```python
from build123d import *

# Parameters (mm, degrees)
F_3_8_16_TAPPED_HOLE2_REACH  = 90.009
F_3_8_16_TAPPED_HOLE2_BORE_R = 3.96875
CIRPATTERN1_COUNT            = 6


with BuildPart() as part:
    # Sketch2 → Revolve1 (revolve)
    with BuildSketch(Plane.XY, mode=Mode.PRIVATE) as revolve1_sk:
        Polygon((-34.8996, 40.689305596), (-25.4, 40.689305596), (-25.4, 4.857627196), (-34.8996, 4.857627196), (-34.8996, 28.497305596), (-32.8676, 28.497305596), (-32.8676, 32.053305596), (-34.8996, 32.053305596), (-34.8996, 34.593305596), (-32.8676, 34.593305596), (-32.8676, 38.149305596), (-34.8996, 38.149305596), align=None)
    revolve(revolve1_sk.sketch.rotate(Axis((0, 0, 0), (0, 1, 0)), 270), axis=Axis((0, 0, 0), (0, 1, 0)))

    # 3/8-16 Tapped Hole2 bore → 3/8-16 Tapped Hole2 (cut, up to next)
    with BuildSketch(Plane(origin=(34.8996, 0, 0), x_dir=(0, 0, -1), z_dir=(1, 0, 0)), mode=Mode.PRIVATE) as f_3_8_16_tapped_hole2_sk1:
        with Locations((0, 17.372080196)):
            Circle(F_3_8_16_TAPPED_HOLE2_BORE_R)
    f_3_8_16_tapped_hole2_tool1 = extrude(f_3_8_16_tapped_hole2_sk1.sketch, amount=-F_3_8_16_TAPPED_HOLE2_REACH, mode=Mode.PRIVATE) & part.part
    f_3_8_16_tapped_hole2 = f_3_8_16_tapped_hole2_tool1.solids().sort_by_distance((34.8996, 17.37208, 0))[0]
    add(f_3_8_16_tapped_hole2, mode=Mode.SUBTRACT)

    # CirPattern1: 3/8-16 Tapped Hole2 ×6 about axis
    cirpattern1_axis = Axis((0, 40.689305596, 0), (0, -1, 0))
    for i in range(1, CIRPATTERN1_COUNT):
        add(f_3_8_16_tapped_hole2.rotate(cirpattern1_axis, i * 360 / CIRPATTERN1_COUNT), mode=Mode.SUBTRACT)


solid = part.part
```
Geometry check sheet. Reference: the model listing, model coordinates, mm. A direction names the side the tool comes from. Round coordinates to 2 decimals unless told otherwise and drop trailing zeros. Order: outer loops, then holes, each group sorted by start corner. A loop starts at its lowest first (then second) coordinate and runs counter-clockwise, first axis right, second up. Notation, with made-up numbers: M 38.25,-30 L 94.25,-30 A9 ccw 94.25,-17 Z; hole C 9.5,-39.75 d10. An arc over 180 degrees is marked long. Write item = value, one per line.
Q1. Scan lines: line 1 (Y direction, x = -26.75, z = 0); line 2 (Z direction, x = 30, y = 18); line 3 (Z direction, x = 17, y = 19.5). Record each from-to range of solid material in increasing order.
Answer block:
line_1 = 4.86 to 13.4, 21.34 to 40.69
line_2 = -17.83 to -3.92, 3.92 to 17.83
line_3 = -22.74 to -18.87, 18.87 to 22.74
Q2. Section check A-A (y = 16.5). Enter the section's corners in (x, z), plus the area to 3 significant figures.
Answer block:
outline = M -34.68,-3.87 A34.9 ccw -20.7,-28.1 L -15.9,-19.8 A25.4 cw -25.1,-3.87 Z; M -34.68,3.87 L -25.1,3.87 A25.4 cw -15.9,19.8 L -20.7,28.1 A34.9 ccw Z; M -13.99,-31.97 A34.9 ccw 13.99,-31.97 L 9.2,-23.68 A25.4 cw -9.2,-23.68 Z; M -13.99,31.97 L -9.2,23.68 A25.4 cw 9.2,23.68 L 13.99,31.97 A34.9 ccw Z; M 15.9,-19.8 L 20.7,-28.1 A34.9 ccw 34.68,-3.87 L 25.1,-3.87 A25.4 cw Z; M 15.9,19.8 A25.4 cw 25.1,3.87 L 34.68,3.87 A34.9 ccw 20.7,28.1 Z
area = 1,360 mm^2
Q3. Release check for a two-part mould opening along Y. For faces 3 (the cylindrical face through (-15.479, 21.307, 25.777)), 4 (the cylindrical face through (30.962, 33.341, -16.104)), 5 (the flat face through (26, 4.858, 2)), 6 (the flat face through (21, 38.149, 26)) record: released by +Y, released by -Y, zero draft, split by the parting line, or undercut.
Answer block:
face_3 = undercut
face_4 = zero draft
face_5 = released by -Y
face_6 = undercut
Q4. Set-up check for faces 1 (the cylindrical face through (-7.629, 22.523, -24.227)), 2 (the flat face through (26, 34.593, -21)): record each of +Z, -Z, +X, -X, +Y, -Y from which the full face is reachable in a straight line by a thin tool's end or side.
Answer block:
face_1 = +Y, -Y
face_2 = none
Q5. Depth check by flat-ended pin: pin 1 Ø1.5 at (y, z) = (32.5, -8) entering from +X; pin 2 Ø21 at (x, z) = (-6, 3) entering from +Y; pin 3 Ø10 at (x, y) = (-26.5, 22.5) entering from +Z; pin 4 Ø4 at (x, y) = (22, 11.5) entering from -Z. Enter the tip coordinate at first touch or a pass-through.
Answer block:
pin_1 = 34.14
pin_2 = through
pin_3 = 27.49
pin_4 = -28.6
Q6. Section check C-C (x = 0). Enter the section's corners in (y, z), plus the area to 3 significant figures.
Answer block:
outline = M 4.86,-34.9 L 28.5,-34.9 L 28.5,-32.87 L 32.05,-32.87 L 32.05,-34.9 L 34.59,-34.9 L 34.59,-32.87 L 38.15,-32.87 L 38.15,-34.9 L 40.69,-34.9 L 40.69,-25.4 L 4.86,-25.4 Z; M 4.86,25.4 L 40.69,25.4 L 40.69,34.9 L 38.15,34.9 L 38.15,32.87 L 34.59,32.87 L 34.59,34.9 L 32.05,34.9 L 32.05,32.87 L 28.5,32.87 L 28.5,34.9 L 4.86,34.9 Z
area = 652 mm^2
Q7. Section check B-B (z = 0). Give the number of separate pieces and of enclosed holes in the cut face, plus the area to 3 significant figures.
Answer block:
separate_pieces = 4
enclosed_holes = 0
area = 501 mm^2
Q8. Section check D-D (z = 18.5). Enter the section's corners in (x, y), plus the area to 3 significant figures.
Answer block:
outline = M -29.59,4.86 L -17.4,4.86 L -17.4,40.69 L -29.59,40.69 L -29.59,38.15 L -27.17,38.15 L -27.17,34.59 L -29.59,34.59 L -29.59,32.05 L -27.17,32.05 L -27.17,28.5 L -29.59,28.5 Z; M 17.4,4.86 L 29.59,4.86 L 29.59,28.5 L 27.17,28.5 L 27.17,32.05 L 29.59,32.05 L 29.59,34.59 L 27.17,34.59 L 27.17,38.15 L 29.59,38.15 L 29.59,40.69 L 17.4,40.69 Z
area = 839 mm^2
